Read the model definition and answer for the solid it produces. Units are mm, in the model's axes. Round coordinates to 2 decimals unless told otherwise and drop trailing zeros. Order: outer loops, then holes, each group sorted by start corner. A loop starts at its lowest first (then second) coordinate and runs counter-clockwise, first axis right, second up. Notation, with made-up numbers: (80, -29) - (119, -29) arc R29 ccw to (119, -4) - close; hole circle Ø9 at (63.5, 64). An arc over 180 degrees is marked (long way). One line per question, with ' | ' between items. Start each with the question number.
1) The part is cut by section B-B, the plane x = 23. Give the vertices of the cut face in (y, z), plus the area to 3 significant figures.
2) Straight lines are drawn through the part: line 1 (X direction, y = 73.75, z = -24.5); line 2 (Z direction, x = 21.5, y = 73.8); line 3 (X direction, y = 73.55, z = -25.5). For each, find the intervals that lie inside material, in ascending order. Write a range as from..to.
3) The part is cut by section C-C, the plane z = -23.75. Give the vertices of the cut face in (x, y).
from build123d import *

# Parameters (mm, degrees)
BOX012_W          = 20
BOX012_H          = 20
BOX012_DEPTH      = 20
BOX011_W          = 8.6
BOX011_H          = 14
BOX011_DEPTH      = 7.6
CYLINDER021_R     = 4.3
CYLINDER021_DEPTH = 10
CYLINDER020_R     = 4.3
CYLINDER020_DEPTH = 10


with BuildPart() as cube012:
    # Box012 → Box012 (new body)
    with BuildSketch(Plane(origin=(10, 53.4, -39), x_dir=(1, 0, 0), z_dir=(0, 0, 1))):
        with Locations((10, 10)):
            Rectangle(BOX012_W, BOX012_H)
    extrude(amount=BOX012_DEPTH)


with BuildPart() as cube011:
    # Box011 → Box011 (new body)
    with BuildSketch(Plane(origin=(17.7, 59, -33.3), x_dir=(1, 0, 0), z_dir=(0, 0, 1))):
        with Locations((4.3, 7)):
            Rectangle(BOX011_W, BOX011_H)
    extrude(amount=BOX011_DEPTH)


with BuildPart() as cylinder021:
    # Cylinder021 → Cylinder021 (new body)
    with BuildSketch(Plane(origin=(22, 73, -26), x_dir=(1, 0, 0), z_dir=(0, -1, 0))):
        Circle(CYLINDER021_R)
    extrude(amount=CYLINDER021_DEPTH)


with BuildPart() as obj1:
    # Cylinder020 → Cylinder020 (new body)
    with BuildSketch(Plane(origin=(22, 73, -33), x_dir=(1, 0, 0), z_dir=(0, -1, 0))):
        Circle(CYLINDER020_R)
    extrude(amount=CYLINDER020_DEPTH)

    # Fusion021: union Cube011, Cylinder021
    add(cube011.part)
    add(cylinder021.part)


with BuildPart() as obj1_1:
    # Fusion021 placement: moved
    add(obj1.part.moved(Location((0, 1, 0))))

    # Cut007002: cut Cube012
    add(cube012.part, mode=Mode.SUBTRACT)


solid = obj1_1.part
Values:
1) outline: (73.4, -37.18) - (74, -37.18) - (74, -21.82) - (73.4, -21.82) - close | area: 9.22 mm^2
2) line 1: x = 17.97..26.03 | line 2: z = -37.27..-21.73 | line 3: x = 17.73..26.27
3) outline: (18.34, 73.4) - (25.66, 73.4) - (25.66, 74) - (18.34, 74) - close
